Could you check a few things on this drawing? It's one solid part, dimensions in mm from its lowest x, y, z. Round coordinates to 2 decimals unless told otherwise and drop trailing zeros. Write each loop counter-clockwise with the first axis right and the second up, starting at its lowest first coordinate (ties: lowest second). Pieces come first, ordered by that corner, then holes. Notation, with made-up numbers: (35, 0) -> (44, 0) arc R10 cw to (44, 6) -> close; hole circle Ø9 at (-15.75, -28.5). An arc over 180 degrees is marked (long way). Answer in a Markdown table with one row per item.
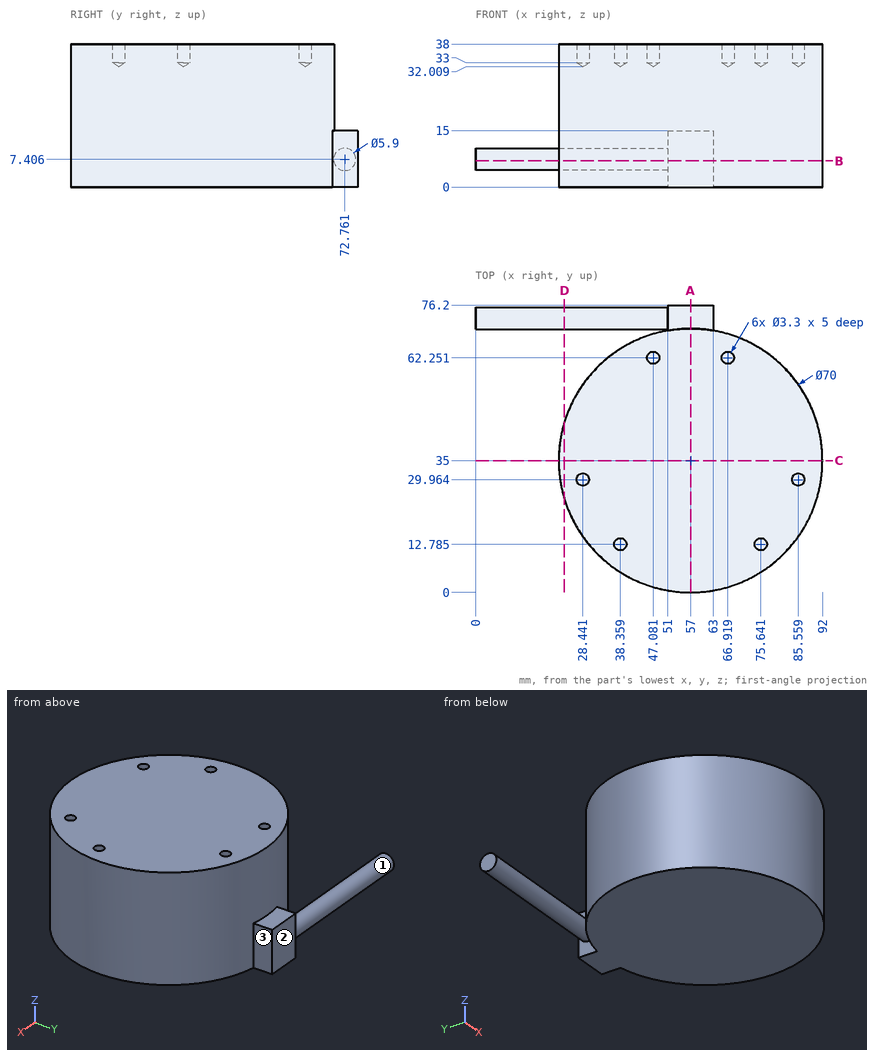
1) I want a section at B-B, the plane z = 7. List the corners of the cut face in (x, y) for me, and give its area (3 significant figures).
Response:
| item | result |
|---|---|
| outline | (0, 69.84) -> (51, 69.84) -> (51, 69.48) arc R35 ccw (long way) to (63, 69.48) -> (63, 76.2) -> (51, 76.2) -> (51, 75.68) -> (0, 75.68) -> close |
| area | 4,220 mm^2 |
2) I want a section at D-D, the plane x = 23.5. List the corners of the cut face in (y, z) for me, and give its area (3 significant figures).
Response:
| item | result |
|---|---|
| outline | (24.86, 0) -> (45.14, 0) -> (45.14, 38) -> (24.86, 38) -> close; circle Ø5.9 at (72.76, 7.41) |
| area | 798 mm^2 |
3) We'd pull the mould along Y, two halves only. Please class the marked faces 1, 2 and 3: +Y half, -Y half, draft (parallel to the pull), parting line (faces both ways), or undercut.
Response:
| item | result |
|---|---|
| face 1 | undercut |
| face 2 | +Y half |
| face 3 | draft |
4) I want a section at A-A, the plane x = 57. List the corners of the cut face in (y, z) for me.
Response:
| item | result |
|---|---|
| outline | (0, 0) -> (76.2, 0) -> (76.2, 15) -> (70, 15) -> (70, 38) -> (0, 38) -> close |
5) For pin 1 (12 mm diameter, centred on x = 37.5, z = 31, fed in from +Y); pin 2 (5.5 mm diameter, centred on x = 58.5, y = 73, fed in from +Z); pin 3 (3.5 mm diameter, centred on y = 73, z = 7, fed in from +X), each with a flat end and sliding along its axis, tell me the tip position at first contact or that it passes through.
Response:
| item | result |
|---|---|
| pin 1 | stops at y = 67.29 |
| pin 2 | stops at z = 15 |
| pin 3 | stops at x = 63 |
6) I want a section at C-C, the plane y = 35. List the corners of the cut face in (x, z) for me.
Response:
| item | result |
|---|---|
| outline | (22, 0) -> (92, 0) -> (92, 38) -> (22, 38) -> close |
7) I need wall thicknesses on line 1 (Z direction, x = 12, y = 72.5) (1 decimal); line 2 (X direction, y = 59, z = 18) (1 decimal); line 3 (Y direction, x = 78.5, z = 25.5). Which ranges of each line are inside material? Lowest first, please. Write a range as [from, to].
Response:
| item | result |
|---|---|
| line 1 | z = [4.5, 10.3] |
| line 2 | x = [31.5, 82.5] |
| line 3 | y = [7.38, 62.62] |
